Could you check a few things on this drawing? It's one solid part, dimensions in mm from its lowest x, y, z. Give positions to 0.01 mm unless a question says otherwise; leave off trailing zeros. Loops run counter-clockwise (first coordinate to the right, second up) from the corner with the lowest first, then second, coordinate; pieces in that order, holes last.
1. Imagine slicing it at A-A (z = 38.1). List the corners of the cut face in (x, y) for me (1 decimal).
2. Imagine slicing it at B-B (y = 1.8). List the corners of the cut face in (x, z) for me (1 decimal).
3. Imagine slicing it at D-D (z = 63.5). List the corners of the cut face in (x, y) for me.
4. Imagine slicing it at C-C (z = 22). List the corners of the cut face in (x, y) for me, plus the area to 3 significant figures.
5. I need wall thicknesses on line 1 along X through (y, z) = (3.95, 63); line 2 along X through (y, z) = (2.1, 38.1) (1 decimal); line 3 along Z through (x, y) = (54.5, 0.3). Which ranges of each line are inside material? Lowest first, please.
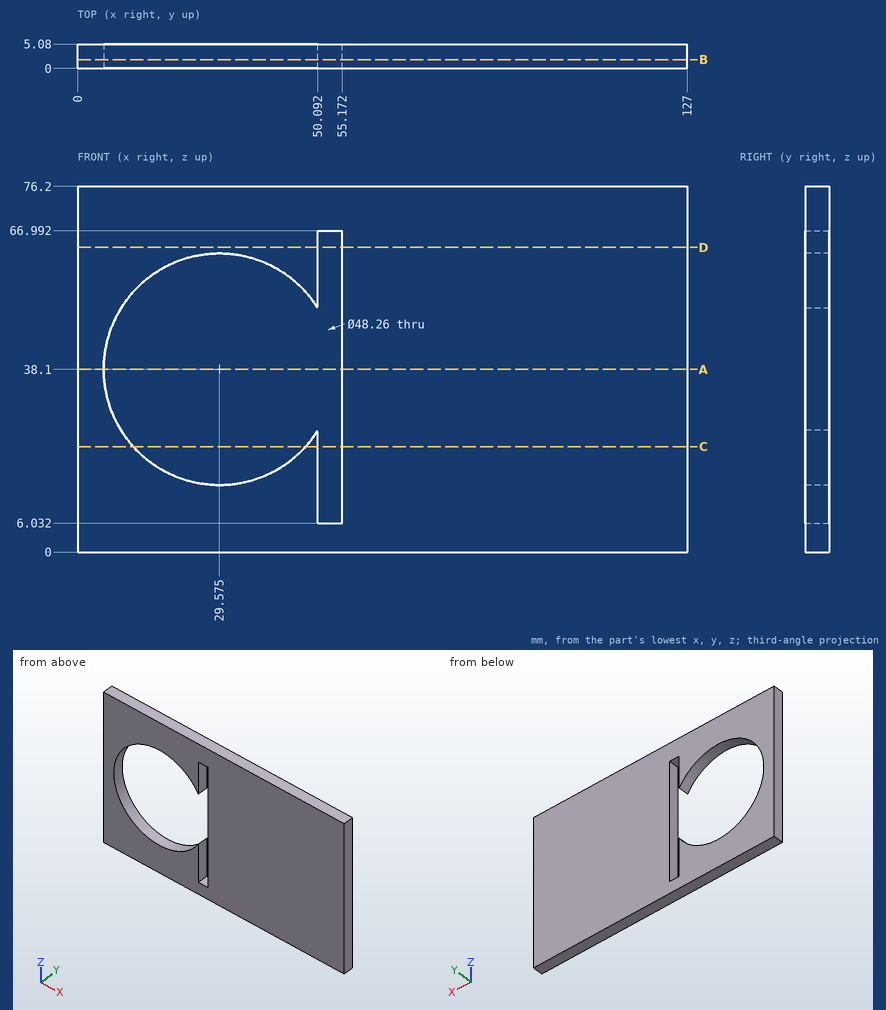
Derived:
1. outline: (0, 0) - (5.4, 0) - (5.4, 5.1) - (0, 5.1) - close; (55.2, 0) - (127, 0) - (127, 5.1) - (55.2, 5.1) - close
2. outline: (0, 0) - (127, 0) - (127, 76.2) - (0, 76.2) - close; hole (50.1, 6) - (55.2, 6) - (55.2, 67) - (50.1, 67) - (50.1, 50.8) arc R24.1 ccw (long way) to (50.1, 25.4) - close
3. outline: (0, 0) - (50.09, 0) - (50.09, 5.08) - (0, 5.08) - close; (55.17, 0) - (127, 0) - (127, 5.08) - (55.17, 5.08) - close
4. outline: (0, 0) - (11.6, 0) - (11.6, 5.08) - (0, 5.08) - close; (47.55, 0) - (50.09, 0) - (50.09, 5.08) - (47.55, 5.08) - close; (55.17, 0) - (127, 0) - (127, 5.08) - (55.17, 5.08) - close
4. area: 437 mm2
5. line 1: x = 0 to 50.09, 55.17 to 127
5. line 2: x = 0 to 5.4, 55.2 to 127
5. line 3: z = 0 to 6.03, 66.99 to 76.2
